Job drawing, mm, ordinate dimensions from the low corner. One solid piece. A direction names the side the tool comes from. Coordinates: 2 decimals unless noted, no trailing zeros. Order: outer loops, then holes, each group sorted by start corner. A loop starts at its lowest first (then second) coordinate and runs counter-clockwise, first axis right, second up. Notation, with made-up numbers: (29, 18) - (33, 18) arc R24 cw to (33, 51) - close; hole circle Ø1 at (88, 34.5). An arc over 180 degrees is marked (long way). Use one line per item in the form item = value.
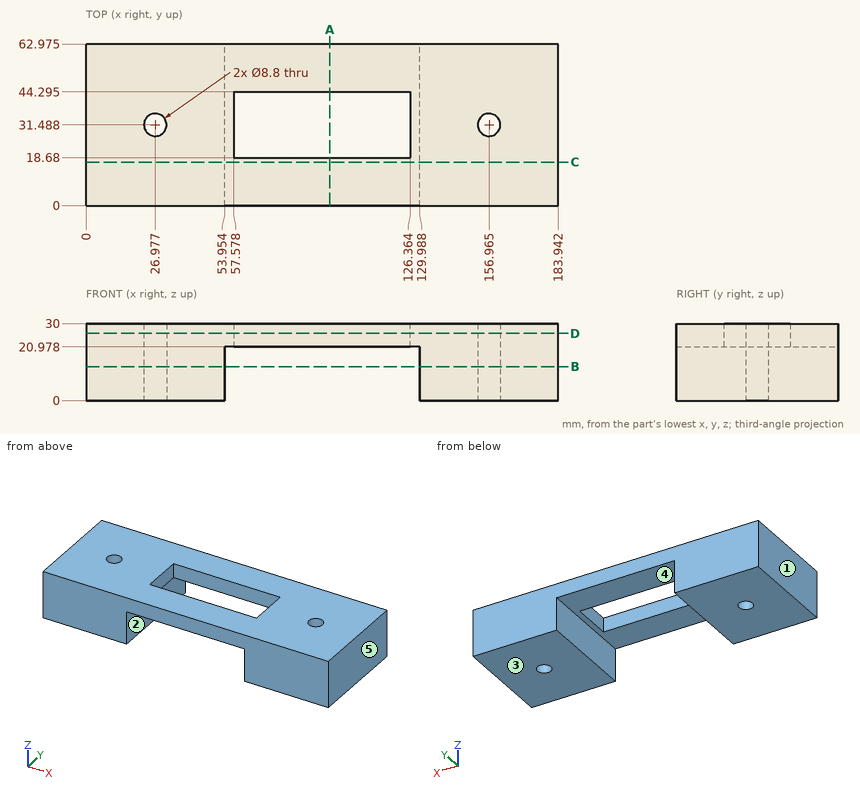
Item 1: Drill centre lines: line 1 (Y direction, x = 122, z = 26.75) (1 decimal); line 2 (X direction, y = 27, z = 24.25); line 3 (X direction, y = 15.5, z = 12). Where is each one in solid material? Low to high. Write a range as [from, to].
Derived:
line_1 = [0, 18.7], [44.3, 63]
line_2 = [0, 57.58], [126.36, 183.94]
line_3 = [0, 53.95], [129.99, 183.94]
Item 2: Cut at A-A, the plane x = 95. Write the cut outline in (y, z) (1 decimal), plus the area to 3 significant figures.
Derived:
outline = (0, 21) - (18.7, 21) - (18.7, 30) - (0, 30) - close; (44.3, 21) - (63, 21) - (63, 30) - (44.3, 30) - close
area = 337 mm²
Item 3: 3-axis set-ups, long thin cutter, end or side, ignore diameter. For the marked faces 1 and 2: which of +Z, -Z, +X, -X, +Y, -Y reach the whole face in a straight line?
Derived:
face_1 = +Z, -Z, -X, +Y, -Y
face_2 = -Z, +Y, -Y
Item 4: Drop flat-ended pins along their axis: pin 1 (12 mm diameter, centred on x = 46.5, y = 52.5, fed in from -Z); pin 2 (19 mm diameter, centred on x = 92, y = 45.5, fed in from -Z). Give the stop position or say it passes through.
Derived:
pin_1 = 0
pin_2 = 20.98
Item 5: Cut at C-C, the plane y = 17. Write the cut outline in (x, z).
Derived:
outline = (0, 0) - (53.95, 0) - (53.95, 20.98) - (129.99, 20.98) - (129.99, 0) - (183.94, 0) - (183.94, 30) - (0, 30) - close
Item 6: Cut at D-D, the plane z = 26.25. Write the cut outline in (x, y) (1 decimal).
Derived:
outline = (0, 0) - (183.9, 0) - (183.9, 63) - (0, 63) - close; hole circle Ø8.8 at (27, 31.5); hole (57.6, 18.7) - (126.4, 18.7) - (126.4, 44.3) - (57.6, 44.3) - close; hole circle Ø8.8 at (157, 31.5)
Item 7: Cut at B-B, the plane z = 13.25. Write the cut outline in (x, y) (1 decimal), plus the area to 3 significant figures.
Derived:
outline = (0, 0) - (54, 0) - (54, 63) - (0, 63) - close; (130, 0) - (183.9, 0) - (183.9, 63) - (130, 63) - close; hole circle Ø8.8 at (27, 31.5); hole circle Ø8.8 at (157, 31.5)
area = 6,670 mm²
Item 8: Two-plate mould, pull along X, no slides. Class the marked faces 3, 4 and 5: +X half, -X half, draft (parallel to the pull), parting line (faces both ways), or undercut.
Derived:
face_3 = draft
face_4 = undercut
face_5 = +X half
